```python
from build123d import *

# Parameters (mm, degrees)
F0_W     = 150
F0_H     = 50
F0_W_2   = 144
F0_H_2   = 44
F1_DEPTH = 45
F3_DEPTH = 53.9
F4_R     = 5


with BuildPart() as f1:
    # F0 (on Top) → F1 (new body)
    with BuildSketch(Plane.XY):
        Rectangle(F0_W, F0_H)
        Rectangle(F0_W_2, F0_H_2, mode=Mode.SUBTRACT)
    extrude(amount=F1_DEPTH)

    # F2 (on face) → F3 (cut)
    with BuildSketch(Plane.XZ.offset(25)):
        with BuildLine():
            ThreePointArc((-31.312153, 45), (-28.654867, 44.235426), (-26.810258, 42.175533))
            ThreePointArc((-26.810258, 42.175533), (0, 25.354907), (26.810258, 42.175533))
            ThreePointArc((26.810258, 42.175533), (28.654867, 44.235426), (31.312153, 45))
            Line((31.312153, 45), (-31.312153, 45))
        make_face()
    extrude(amount=-F3_DEPTH, mode=Mode.SUBTRACT)

    # F4
    f4_edges = [f1.edges().sort_by_distance(p)[0] for p in [
        (-75, 25, 22.5),
        (-75, -25, 22.5),
        (75, 25, 22.5),
        (75, -25, 22.5),
        (-72, -22, 22.5),
        (72, -22, 22.5),
        (72, 22, 22.5),
        (-72, 22, 22.5),
    ]]
    fillet(f4_edges, radius=F4_R)


solid = f1.part
```
Can you work these out from the model? Positions are in its coordinate system, mm. A direction names the side the tool comes from. Round coordinates to 2 decimals unless told otherwise and drop trailing zeros. Order: outer loops, then holes, each group sorted by start corner. A loop starts at its lowest first (then second) coordinate and runs counter-clockwise, first axis right, second up. Notation, with made-up numbers: (76, 36) -> (120, 36) arc R19 ccw to (120, 45) -> close; hole circle Ø10 at (79, 36.25). An arc over 180 degrees is marked (long way). Return JSON: item names as keys, results as strings. Group by question number.
1. Which directions (+Z, -Z, +X, -X, +Y, -Y) give clear straight access to the entire face, cutting with the end or side of a thin tool? Please do faces 4 (the face through (-74, -23, 23)), 5 (the face through (28.6, 23.5, 44.2)), 6 (the face through (-1, -22, 22)).
2. If we section it at C-C, the plane y = 11: Write out the boundary of the cut face in (x, z), then the cut area to 3 significant figures.
3. I need wall thicknesses on line 1 (Y direction, x = 35, z = 10); line 2 (X direction, y = 10, z = 28); line 3 (X direction, y = 21, z = 8). Which ranges of each line are inside material? Lowest first, please. Write a range as [from, to].
4. If we section it at A-A, the plane x = 58.5: Write out the boundary of the cut face in (y, z), then the cut area to 3 significant figures.
5. If we section it at D-D, the plane z = 31.5: Write out the boundary of the cut face in (x, y).
6. If we section it at B-B, the plane z = 6.5: Write out the boundary of the cut face in (x, y).
7. We'd pull the mould along X, two halves only. Please class faces 1 (the face through (72.5, 0.1, 45)), 2 (the face through (28.6, -23.5, 44.2)), 3 (the face through (-74, 23, 23)): released by +X, released by -X, zero draft, split by the parting line, or undercut.
Output values:
{
 "1": {"face 4": "+Z, -Z, -X, -Y", "face 5": "+Z, +Y, -Y", "face 6": "+Z, -Z"},
 "2": {"outline": "(-75, 0) -> (-72, 0) -> (-72, 45) -> (-75, 45) -> close; (72, 0) -> (75, 0) -> (75, 45) -> (72, 45) -> close", "area": "270 mm²"},
 "3": {"line 1": "[-25, -22], [22, 25]", "line 2": "[-75, -72], [72, 75]", "line 3": "[-74.9, -70], [70, 74.9]"},
 "4": {"outline": "(-25, 0) -> (-22, 0) -> (-22, 45) -> (-25, 45) -> close; (22, 0) -> (25, 0) -> (25, 45) -> (22, 45) -> close", "area": "270 mm²"},
 "5": {"outline": "(-75, -20) arc R5 ccw to (-70, -25) -> (-18.12, -25) -> (-18.12, -22) -> (-67, -22) arc R5 cw to (-72, -17) -> (-72, 17) arc R5 cw to (-67, 22) -> (-18.12, 22) -> (-18.12, 25) -> (-70, 25) arc R5 ccw to (-75, 20) -> close; (18.12, -25) -> (70, -25) arc R5 ccw to (75, -20) -> (75, 20) arc R5 ccw to (70, 25) -> (18.12, 25) -> (18.12, 22) -> (67, 22) arc R5 cw to (72, 17) -> (72, -17) arc R5 cw to (67, -22) -> (18.12, -22) -> close"},
 "6": {"outline": "(-75, -20) arc R5 ccw to (-70, -25) -> (70, -25) arc R5 ccw to (75, -20) -> (75, 20) arc R5 ccw to (70, 25) -> (-70, 25) arc R5 ccw to (-75, 20) -> close; hole (-72, -17) arc R5 ccw to (-67, -22) -> (67, -22) arc R5 ccw to (72, -17) -> (72, 17) arc R5 ccw to (67, 22) -> (-67, 22) arc R5 ccw to (-72, 17) -> close"},
 "7": {"face 1": "zero draft", "face 2": "undercut", "face 3": "released by -X"}
}
